Autodesk Inventor part; units mm, degrees
ref_plane "YZ Plane" through (0, 0, 0) normal (1, 0, 0) x (0, 1, 0)
ref_plane "XZ Plane" through (0, 0, 0) normal (0, 1, 0) x (-1, 0, 0)
ref_plane "XY Plane" through (0, 0, 0) normal (0, 0, 1) x (1, 0, 0)
sketch "Sketch1" plane through (0, 0, 0) normal (0, 0, 1) x (1, 0, 0)
  line L0 (0, 0) -> (50.8, 0)
  line L1 (0, 0) -> (0, 63.5)
  line L2 (0, 63.5) -> (6.35, 63.5)
  line L3 (6.35, 63.5) -> (6.35, 6.35)
  line L4 (6.35, 6.35) -> (50.8, 6.35)
  line L5 (50.8, 6.35) -> (50.8, 0)
  dimension "d0" = 50.8
  dimension "d1" = 63.5
  dimension "d2" = 6.35
  dimension "d3" = 6.35
extrude "Extrusion1" add sketch "Sketch1" along normal mid plane 330.2
sketch "Sketch3" plane through (6.35, 6.35, 165.1) normal (1, 0, 0) x (0, 0, -1)
  line L0 (0, 0) -> (0, 57.15)
  line L1 (330.2, 57.15) -> (0, 57.15)
  line L2 (0, 0) -> (91.44, 0)
  line L3 (91.44, 0) -> (91.44, 57.15)
  line L4 (91.44, 57.15) -> (0, 57.15)
  line L5 (0, 57.15) -> (0, 0)
  point P0 (165.1, -6.35)
  dimension "d6" = 91.44
extrude "Extrusion2" cut sketch "Sketch3" against normal through all
properties part number "base"
Can you work these out from the model? Positions are in its coordinate system, mm. A direction names the side the tool comes from. Give positions to 0.01 mm unless a question says otherwise; leave off trailing zeros. Order: outer loops, then holes, each group sorted by start corner. A loop starts at its lowest first (then second) coordinate and runs counter-clockwise, first axis right, second up. Notation, with made-up numbers: M -31.5,9.5 L 12.5,9.5 A12 cw 12.5,32.5 Z; hole C 81.25,34 d7. An arc over 180 degrees is marked long. Use one line per item in the form item = value. Start each with the question number.
Item 1: If we section it at C-C (y = 44): Write out the boundary of the cut face in (x, z), then the cut area to 3 significant figures.
Item 2: Will these pins go through, and if not, where does the flat tip stop? pin 1 Ø4 at (y, z) = (12.5, -47) entering from +X; pin 2 Ø3 at (x, y) = (4, 42) entering from +Z.
Item 3: If I drill on line 1 along Y through (x, z) = (45, 73.5); line 2 along Z through (x, y) = (3, 30.5), over which ranges is the centre line in solid material (lowest first)?
Item 4: If we section it at B-B (x = 38): Write out the boundary of the cut face in (y, z), then the cut area to 3 significant figures.
Item 5: For faces 1 (the flat face through (3, 35, 73.66)), 2 (the flat face through (6.35, 35, -47)), 3 (the flat face through (0, 31, -39)), which set-ups out of +Z, -Z, +X, -X, +Y, -Y let a thin tool reach every point of the face, with its end or its side?
Item 6: If we section it at A-A (z = -71.5): Write out the boundary of the cut face in (x, y).
Outcome:
q1.outline = M 0,-165.1 L 6.35,-165.1 L 6.35,73.66 L 0,73.66 Z
q1.area = 1,520 mm2
q2.pin_1 = 6.35
q2.pin_2 = 73.66
q3.line_1 = 0 to 6.35
q3.line_2 = -165.1 to 73.66
q4.outline = M 0,-165.1 L 6.35,-165.1 L 6.35,165.1 L 0,165.1 Z
q4.area = 2,100 mm2
q5.face_1 = +Z, +X, -X, +Y
q5.face_2 = +Z, -Z, +X, +Y
q5.face_3 = +Z, -Z, -X, +Y, -Y
q6.outline = M 0,0 L 50.8,0 L 50.8,6.35 L 6.35,6.35 L 6.35,63.5 L 0,63.5 Z
